Read the model definition and answer for the solid it produces. Units are mm, in the model's axes. Face numbers are marked on the shaded views. A direction names the side the tool comes from. Give positions to 0.01 mm unless a question says otherwise; leave off trailing zeros. Write each loop counter-clockwise with the first axis right and the second up, starting at its lowest first coordinate (ties: lowest second). Pieces come first, ordered by that corner, then holes. Notation, with made-up numbers: (44, -20.75) -> (96, -20.75) arc R18 ccw to (96, 5.25) -> close; hole circle Ø4 at (11.5, -23.5). An arc over 180 degrees is marked (long way). Write item = value, one per line.
from build123d import *
from build123d.topology import SkipClean

# Parameters (mm, degrees)
SKETCH1_R               = 22.5
SKETCH1_R_2             = 3.15
SKETCH1_R_3             = 1.65
BOSS_EXTRUDE1_DEPTH     = 2
BOSS_EXTRUDE2_START     = 9
SKETCH2_R               = 8.15
SKETCH2_R_2             = 3.15
BOSS_EXTRUDE2_DEPTH     = 9
CUT_EXTRUDE1_DEPTH      = 53.886222213
CUT_EXTRUDE1_DEPTH_BACK = 53.886222213
SKETCH3_W               = 59.321790447
SKETCH3_H               = 68.701430229
BOSS_EXTRUDE4_START     = -11
BOSS_EXTRUDE4_DEPTH     = 11
CUT_EXTRUDE2_DEPTH      = 2.8
CUT_EXTRUDE2_DEPTH_BACK = 2
CUT_EXTRUDE2_START      = -9.55
SKETCH5_R               = 1.5
CUT_EXTRUDE3_DEPTH      = 35.543052847
BOSS_EXTRUDE3_START     = 3
SKETCH6_R               = 2.9
BOSS_EXTRUDE3_DEPTH     = 3


# Read off the part's stored shape, not the designer's step: Boss-Extrude4
with BuildPart() as part:
    # Sketch1 → Boss-Extrude1 (new body)
    with BuildSketch(Plane.XY):
        with Locations((-12.05, 16)):
            Circle(SKETCH1_R)
        with Locations((-12.05, 16)):
            Circle(SKETCH1_R_2, mode=Mode.SUBTRACT)
        with Locations((-29.25, 16)):
            Circle(SKETCH1_R_3, mode=Mode.SUBTRACT)
        with Locations((5.15, 16)):
            Circle(SKETCH1_R_3, mode=Mode.SUBTRACT)
    extrude(amount=BOSS_EXTRUDE1_DEPTH)

    # Sketch2 → Boss-Extrude2 (add)
    with SkipClean():  # the faces are left unmerged after this step: merging them gives an invalid solid
        with BuildSketch(Plane(origin=(0, 0, 0), x_dir=(-1, 0, 0), z_dir=(0, 0, -1)).offset(BOSS_EXTRUDE2_START)):
            with Locations(Location((12.05, 16, 0), (0, 0, 180))):
                Circle(SKETCH2_R)
            with Locations((12.05, 16)):
                Circle(SKETCH2_R_2, mode=Mode.SUBTRACT)
        extrude(amount=-BOSS_EXTRUDE2_DEPTH)

    # Sketch3 → Cut-Extrude1 (cut, two sides: drawn at the far end of the back side and taken through both)
    with BuildSketch(Plane.XY.offset(2).offset(-CUT_EXTRUDE1_DEPTH_BACK)):
        with Locations((-10.056838751, 16.22852839)):
            Rectangle(SKETCH3_W, SKETCH3_H)
        with BuildLine():
            Line((-30.128197674, 10.773264035), (-13.400436047, 7.962660734))
            ThreePointArc((-13.400436047, 7.962660734), (-3.9, 16), (-13.400436047, 24.037339266))
            Line((-13.400436047, 24.037339266), (-30.128197674, 21.226735965))
            ThreePointArc((-30.128197674, 21.226735965), (-34.55, 16), (-30.128197674, 10.773264035))
        make_face(mode=Mode.SUBTRACT)
    extrude(amount=CUT_EXTRUDE1_DEPTH + CUT_EXTRUDE1_DEPTH_BACK, mode=Mode.SUBTRACT)

    # Boss-Extrude4 outline → Boss-Extrude4 (add)
    with BuildSketch(Plane.XY.offset(2).offset(BOSS_EXTRUDE4_START)):
        with BuildLine():
            ThreePointArc((-9.55, 14.08362321), (-8.9, 16), (-9.55, 17.91637679))
            Line((-9.55, 17.91637679), (-9.55, 14.08362321))
        make_face()
    extrude(amount=BOSS_EXTRUDE4_DEPTH)

    # Sketch4 → Cut-Extrude2 (cut, two sides: drawn at the far end of the back side and taken through both)
    with BuildSketch(Plane(origin=(0, 0, 0), x_dir=(0, 0, -1), z_dir=(1, 0, 0)).offset(CUT_EXTRUDE2_START - CUT_EXTRUDE2_DEPTH_BACK)):
        Polygon((-0.5, 17.675), (-0.5, 14.325), (2.401185103, 12.65), (5.302370205, 14.325), (5.302370205, 17.675), (2.401185103, 19.35), align=None)
    extrude(amount=CUT_EXTRUDE2_DEPTH + CUT_EXTRUDE2_DEPTH_BACK, mode=Mode.SUBTRACT)

    # Sketch5 → Cut-Extrude3 (cut, through all)
    with BuildSketch(Plane.ZY.offset(11.55)):
        with Locations((-2.401185103, 16)):
            Circle(SKETCH5_R)
    extrude(amount=-CUT_EXTRUDE3_DEPTH, mode=Mode.SUBTRACT)

    # Sketch6 → Boss-Extrude3 (add)
    with BuildSketch(Plane(origin=(0, 0, 0), x_dir=(-1, 0, 0), z_dir=(0, 0, -1)).offset(BOSS_EXTRUDE3_START)):
        with BuildLine():
            Line((30.128197674, 21.226735965), (13.400436047, 24.037339266))
            ThreePointArc((13.400436047, 24.037339266), (20.2, 16), (13.400436047, 7.962660734))
            Line((13.400436047, 7.962660734), (30.128197674, 10.773264035))
            ThreePointArc((30.128197674, 10.773264035), (34.55, 16), (30.128197674, 21.226735965))
        make_face()
        with Locations((29.25, 16)):
            Circle(SKETCH6_R, mode=Mode.SUBTRACT)
    extrude(amount=-BOSS_EXTRUDE3_DEPTH)


solid = part.part
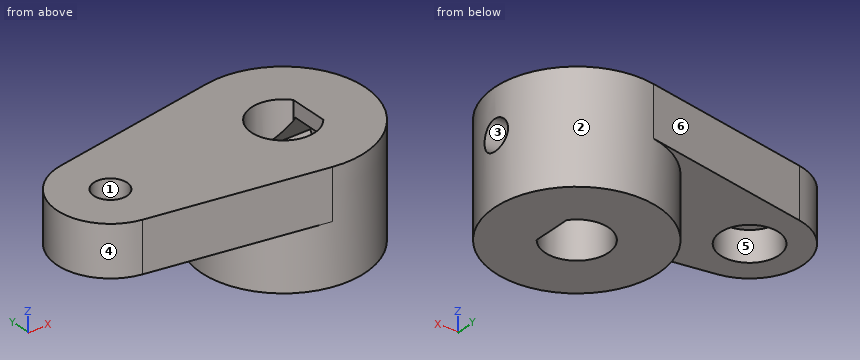
(1) The part is cut by section D-D on y = 20. Determine the outline of the cut face in (x, z), plus the area to 3 significant figures.
Checks:
outline = (-32.73, -3) -> (-19.15, -3) -> (-19.15, -9) -> (-4.95, -9) -> (-4.95, 2) -> (-32.73, 2) -> close
area = 224 mm²
(2) For a pull along X with two mould halves and no side action, classify the marked faces 1, 2, 3 and 4 as released by +X, released by -X, zero draft, split by the parting line, or undercut.
Checks:
face_1 = undercut
face_2 = split by the parting line
face_3 = zero draft
face_4 = released by -X
(3) The part is cut by section B-B on x = -12.05. Determine the outline of the cut face in (y, z).
Checks:
outline = (7.85, -9) -> (12.85, -9) -> (12.85, 2) -> (7.85, 2) -> close; (19.15, -9) -> (24.15, -9) -> (24.15, 2) -> (19.15, 2) -> close
(4) A tool of negligible diameter and unlimited length cuts with its end or side. For the marked faces 5 and 6, from which of +Z, -Z, +X, -X, +Y, -Y can it reach the whole face along a straight path? Write none if from no direction.
Checks:
face_5 = -Z
face_6 = +Z, -Z, -X, +Y
(5) The part is cut by section A-A on y = 16. Determine the outline of the cut face in (x, z).
Checks:
outline = (-34.55, -3) -> (-32.15, -3) -> (-32.15, 0) -> (-30.9, 0) -> (-30.9, 2) -> (-34.55, 2) -> close; (-27.6, 0) -> (-26.35, 0) -> (-26.35, -3) -> (-20.2, -3) -> (-20.2, -9) -> (-15.2, -9) -> (-15.2, 2) -> (-27.6, 2) -> close; (-9.55, -9) -> (-3.9, -9) -> (-3.9, -3.9) -> (-6.75, -3.9) -> (-6.75, -5.3) -> (-9.55, -5.3) -> close; (-9.55, 0.5) -> (-6.75, 0.5) -> (-6.75, -0.9) -> (-3.9, -0.9) -> (-3.9, 2) -> (-9.55, 2) -> close
(6) The part is cut by section C-C on z = -4.25. Determine the outline of the cut face in (x, y).
Checks:
outline = circle Ø16.3 at (-12.05, 16); hole (-9.88, 13.72) -> (-6.75, 13.72) -> (-6.75, 18.28) -> (-9.88, 18.28) arc R3.15 ccw (long way) to start
(7) Given P1, Ø5.5, axis at x = -29.25, y = 16, coming from the -Z side; P2, Ø1, axis at x = -27.5, z = 0, coming from the -Y side; P3, Ø2, axis at x = -21.5, y = 13, coming from the -Z side, each flat-ended and moving along its own axis, determine where each tip first touches the part or whether it passes through.
Checks:
P1 = 0
P2 = 10.25
P3 = -3
(8) Consider L1, parallel to Y at x = -12, z = -3.75; L2, parallel to Z at x = -5.25, y = 16; L3, parallel to X at y = 16.5, z = -0.75. Determine where each line is inside the solid, lowest interval first.
Checks:
L1 = 7.85 to 12.85, 19.15 to 24.15
L2 = -9 to -3.9, -0.9 to 2
L3 = -34.53 to -32.11, -26.39 to -15.16, -6.75 to -3.92
